Verification items for the finished model (mm, model axes). A direction names the side the tool comes from. Give positions to 0.01 mm unless a question says otherwise; leave off trailing zeros. Loops run counter-clockwise (first coordinate to the right, second up) from the corner with the lowest first, then second, coordinate; pieces in that order, holes last. Notation, with made-up numbers: (-4.75, 67.25) - (7.25, 67.25) arc R23 ccw to (7.25, 97.25) - close; hole circle Ø4 at (64.5, -27.75). An arc over 180 degrees is marked (long way). One line per item, written item: value. Start each with the question number.
1. Gauge pin test, flat ends, axial feed: pin 1 (6.5 mm diameter, centred on x = -0.2, y = 10.35, fed in from -Z); pin 2 (5.5 mm diameter, centred on x = -0.49, y = -7.32, fed in from +Z); pin 3 (4 mm diameter, centred on x = -17.87, y = 10.64, fed in from +Z); pin 4 (3 mm diameter, centred on x = -0.49, y = -7.32, fed in from +Z). Record the tip position at first contact, or that the pin passes through.
2. Access from +Z, -Z, +X, -X, +Y, -Y to the whole of each face (thin tool, end or side, straight path). Record for faces 4 (the flat face through (-10, 2, 8)), 5 (the cylindrical face through (-17.11, 7.23, 6.48)).
3. Sectioned sample at A-A (z = 7). Record the cut outline in (x, y), plus the area to 3 significant figures.
4. Scan lines: L1, parallel to X at y = 10.5, z = 6; L2, parallel to X at y = 11.75, z = 5.5; L3, parallel to Y at x = -17, z = 7.25. Record each from-to range of solid material in increasing order. Write a range as [from, to].
5. Mould release check, pull along X, two halves, no side actions. Record for faces 1 (the cylindrical face through (0.562, 6.936, 6.479)), 2 (the flat face through (-10, 16.661, 4)), 3 (the flat face through (-59.18, 1, 4)): pulls with the +X half, pulls with the -X half, needs draft (parallel to the pull), parting line crosses it, or undercut.
from build123d import *

# Parameters (mm, degrees)
F0_W     = 100
F0_H     = 30
F1_DEPTH = 8
F3_D     = 7
F3_DEPTH = 3
F3_TIP   = 2.1030121666


with BuildPart() as f1:
    # F0 (on Top) → F1 (new body)
    with BuildSketch(Plane.XY):
        with Locations((-9.1803266555, 1.6609177441)):
            Rectangle(F0_W, F0_H)
        with BuildLine():
            ThreePointArc((-16.4140304677, -7.0306336602), (-19.7862985458, -7.6869463014), (-16.906311934, -5.8138164636))
            ThreePointArc((-16.906311934, -5.8138164636), (-16.5417623897, -6.374321019), (-16.4140304677, -7.0306336602))
        make_face(mode=Mode.SUBTRACT)
        with BuildLine():
            ThreePointArc((1.2612247488, -7.3227860681), (-1.1718088909, -8.9339859462), (-1.7055924478, -6.0650675344))
            ThreePointArc((-1.7055924478, -6.0650675344), (0.1942583885, -5.7115861901), (1.2612247488, -7.3227860681))
        make_face(mode=Mode.SUBTRACT)
        with BuildLine():
            ThreePointArc((-16.6550608632, 9.3869030227), (-19.4830779378, 11.3276551961), (-16.1218780598, 10.6446215564))
            ThreePointArc((-16.1218780598, 10.6446215564), (-16.2606781817, 9.9615879167), (-16.6550608632, 9.3869030227))
        make_face(mode=Mode.SUBTRACT)
        with BuildLine():
            ThreePointArc((1.5533771568, 10.3524691484), (0.459689798, 8.7302010704), (-1.4543413769, 9.1356519518))
            ThreePointArc((-1.4543413769, 9.1356519518), (-0.8529354844, 11.9747372265), (1.5533771568, 10.3524691484))
        make_face(mode=Mode.SUBTRACT)
    extrude(amount=F1_DEPTH)

    # F3
    with Locations(Plane.XY.offset(8)):
        with Locations((-0.4887752512, -7.3227860681), (-18.1640304677, -7.0306336602), (-17.8718780598, 10.6446215564), (-0.1966228432, 10.3524691484)):
            Hole(F3_D / 2, depth=F3_DEPTH)
            with Locations((0, 0, -(F3_DEPTH + F3_TIP / 2))):  # 118° drill point
                Cone(0, F3_D / 2, F3_TIP, mode=Mode.SUBTRACT)


solid = f1.part
Results are:
1. pin 1: stops at z = 0
1. pin 2: stops at z = 4.55
1. pin 3: stops at z = 4.1
1. pin 4: passes through
2. face 4: +Z, +X, -X, +Y, -Y
2. face 5: +Z
3. outline: (-59.18, -13.34) - (40.82, -13.34) - (40.82, 16.66) - (-59.18, 16.66) - close; hole circle Ø7 at (-18.16, -7.03); hole circle Ø7 at (-17.87, 10.64); hole circle Ø7 at (-0.49, -7.32); hole circle Ø7 at (-0.2, 10.35)
3. area: 2,850 mm^2
4. L1: x = [-59.18, -21.37], [-14.37, -3.69], [3.3, 40.82]
4. L2: x = [-59.18, -21.19], [-14.55, -3.41], [3.01, 40.82]
4. L3: y = [-13.34, -10.33], [-3.73, 7.25], [14.03, 16.66]
5. face 1: undercut
5. face 2: needs draft
5. face 3: pulls with the -X half
